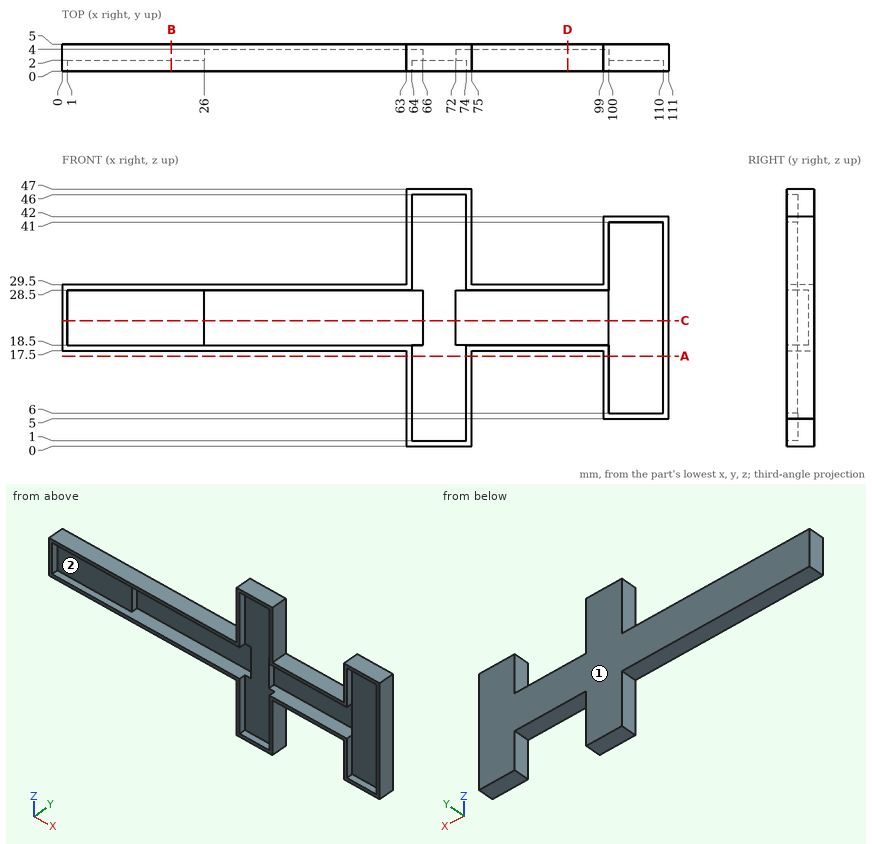
Verification items for this drawing (mm, ordinates from the low corner). Give positions to 0.01 mm unless a question says otherwise; leave off trailing zeros. Loops run counter-clockwise (first coordinate to the right, second up) from the corner with the lowest first, then second, coordinate; pieces in that order, holes last. Notation, with made-up numbers: M 11.25,28 L 55.25,28 A23 cw 55.25,55 Z; hole C 79.5,2.25 d10. An arc over 180 degrees is marked long. Write each question's results on one line, items separated by ' | '.
1) Section check A-A, the plane z = 16.5. Record the boundary of the cut face in (x, y), plus the area to 3 significant figures.
Answers follow:
outline: M 63,0 L 64,0 L 64,2 L 74,2 L 74,0 L 75,0 L 75,5 L 63,5 Z; M 99,0 L 100,0 L 100,2 L 110,2 L 110,0 L 111,0 L 111,5 L 99,5 Z | area: 80.0 mm2
2) Gauge pin test, flat ends, axial feed: pin 1 (0.6 mm diameter, centred on y = 0.5, z = 16, fed in from -X); pin 2 (1.5 mm diameter, centred on x = 85, y = 2, fed in from +Z); pin 3 (6 mm diameter, centred on x = 27, z = 30.5, fed in from -Y); pin 4 (1 mm diameter, centred on x = 27, z = 30.5, fed in from +Y). Record the tip position at first contact, or that the pin passes through.
Answers follow:
pin 1: x = 63 | pin 2: z = 29.5 | pin 3: y = 0 | pin 4: through
3) Section check D-D, the plane x = 92.5. Record the boundary of the cut face in (y, z).
Answers follow:
outline: M 0,17.5 L 5,17.5 L 5,29.5 L 0,29.5 L 0,28.5 L 4,28.5 L 4,18.5 L 0,18.5 Z
4) Release check for a two-part mould opening along Z. For the marked faces 1 and 2 record: +Z half, -Z half, draft (parallel to the pull), parting line (faces both ways), or undercut.
Answers follow:
face 1: draft | face 2: undercut
5) Section check B-B, the plane x = 20. Record the boundary of the cut face in (y, z), plus the area to 3 significant figures.
Answers follow:
outline: M 0,17.5 L 5,17.5 L 5,29.5 L 0,29.5 L 0,28.5 L 2,28.5 L 2,18.5 L 0,18.5 Z | area: 40.0 mm2
6) Thickness scan on line 1 (X direction, y = 0.75, z = 10); line 2 (X direction, y = 3.5, z = 21); line 3 (Z direction, x = 78.5, y = 2.4). Record the ranges inside material, lowest first.
Answers follow:
line 1: 63 to 64, 74 to 75, 99 to 100, 110 to 111 | line 2: 0 to 26, 66 to 72, 100 to 111 | line 3: 17.5 to 18.5, 28.5 to 29.5
7) Section check C-C, the plane z = 23. Record the boundary of the cut face in (x, y).
Answers follow:
outline: M 0,0 L 1,0 L 1,2 L 26,2 L 26,4 L 66,4 L 66,2 L 72,2 L 72,4 L 100,4 L 100,2 L 110,2 L 110,0 L 111,0 L 111,5 L 0,5 Z
